from build123d import *

# Parameters (mm, degrees)
SKETCH1_W       = 30
SKETCH1_H       = 64
BLOCK_DEPTH     = 37.5
BLOCKFILLET_R   = 3
SKETCH2_R       = 5.5
JACKHOLES_DEPTH = 36.5


with BuildPart() as part:
    # Sketch1 → Block (new body)
    with BuildSketch(Plane.YZ):
        Rectangle(SKETCH1_W, SKETCH1_H)
    extrude(amount=BLOCK_DEPTH)

    # BlockFillet
    blockfillet_edges = [part.edges().sort_by_distance(p)[0] for p in [
        (18.75, -15, 32),
        (18.75, 15, 32),
        (18.75, 15, -32),
        (18.75, -15, -32),
    ]]
    fillet(blockfillet_edges, radius=BLOCKFILLET_R)

    # Sketch2 → JackHoles (cut)
    with BuildSketch(Plane(origin=(0, 0, 0), x_dir=(0, -1, 0), z_dir=(-1, 0, 0))):
        with Locations(Location((-3, -20, 0), (0, 0, 90))):
            Circle(SKETCH2_R)
        with Locations(Location((-3, 0, 0), (0, 0, 90))):
            Circle(SKETCH2_R)
        with Locations(Location((-3, 20, 0), (0, 0, 90))):
            Circle(SKETCH2_R)
    extrude(amount=-JACKHOLES_DEPTH, mode=Mode.SUBTRACT)


solid = part.part
Model file for the job. Use its own axes, mm. A direction names the side the tool comes from. Coordinates: 2 decimals unless noted, no trailing zeros. Order: outer loops, then holes, each group sorted by start corner. A loop starts at its lowest first (then second) coordinate and runs counter-clockwise, first axis right, second up. Notation, with made-up numbers: M -40,67 L -25,67 A27 ccw -25,88 Z; hole C 59.5,12.5 d2. An arc over 180 degrees is marked long. Return JSON: item names as keys, results as strings.
1. Saw through at A-A (x = 34.5). Give the cut face in (y, z).
Ans:
{"outline": "M -15,-29 A3 ccw -12,-32 L 12,-32 A3 ccw 15,-29 L 15,29 A3 ccw 12,32 L -12,32 A3 ccw -15,29 Z; hole C 3,-20 d11; hole C 3,0 d11; hole C 3,20 d11"}
2. Saw through at B-B (y = 3). Give the cut face in (x, z).
Ans:
{"outline": "M 0,-32 L 37.5,-32 L 37.5,32 L 0,32 L 0,25.5 L 36.5,25.5 L 36.5,14.5 L 0,14.5 L 0,5.5 L 36.5,5.5 L 36.5,-5.5 L 0,-5.5 L 0,-14.5 L 36.5,-14.5 L 36.5,-25.5 L 0,-25.5 Z"}
3. Flat gauge pin, fed straight in: pin 1 (9 mm diameter, centred on y = 1, z = 19.5, fed in from -X). Where does the tip first touch, or does it go through?
Ans:
{"pin 1": "x = 0"}
4. Saw through at C-C (z = -20). Give the cut face in (x, y), and give its area (4 significant figures).
Ans:
{"outline": "M 0,-15 L 37.5,-15 L 37.5,15 L 0,15 L 0,8.5 L 36.5,8.5 L 36.5,-2.5 L 0,-2.5 Z", "area": "723.5 mm^2"}
5. Pull direction Z, two halves, no side cores. Call faces 3 (the face through (17.99, 0.89, -14.92)), 4 (the face through (19.01, -14.14, -31.1)), 5 (the face through (18, -15, 0)): +Z half, -Z half, draft (parallel to the pull), parting line (faces both ways), or undercut.
Ans:
{"face 3": "undercut", "face 4": "-Z half", "face 5": "draft"}
6. Drill centre lines: probe 1 along Y at (x, z) = (26.5, -20); probe 2 along Z at (x, y) = (36, 0.5); probe 3 along Z at (x, y) = (3, 3.25). Where is each one in solid material? Low to high.
Ans:
{"probe 1": "-15 to -2.5, 8.5 to 15", "probe 2": "-32 to -24.9, -15.1 to -4.9, 4.9 to 15.1, 24.9 to 32", "probe 3": "-32 to -25.49, -14.51 to -5.49, 5.49 to 14.51, 25.49 to 32"}
7. Saw through at D-D (z = -2.5). Give the cut face in (x, y).
Ans:
{"outline": "M 0,-15 L 37.5,-15 L 37.5,15 L 0,15 L 0,7.9 L 36.5,7.9 L 36.5,-1.9 L 0,-1.9 Z"}
8. Tool access for faces 1 (the face through (19.01, 14.14, 31.1)), 2 (the face through (36.5, 3, 20)): list every direction of +Z, -Z, +X, -X, +Y, -Y with a clear straight run to the whole face (end or side of a thin tool).
Ans:
{"face 1": "+Z, +X, -X, +Y", "face 2": "-X"}
